from build123d import *

# Parameters (mm, degrees)
SKETCH2_W                        = 1244.6
SKETCH2_H                        = 69.85
BASE_FLANGE1_DEPTH               = 3.2639
EDGE_FLANGE1_STRIP_W             = 15.5956
EDGE_FLANGE1_STRIP_H             = 3.2639
EDGE_FLANGE1_STRIP_CUT_DEPTH     = 1244.6
EDGE_FLANGE1_STRIP_2_W           = 15.5956
EDGE_FLANGE1_STRIP_2_H           = 3.2639
EDGE_FLANGE1_STRIP_CUT_2_DEPTH   = 1244.6
EDGE_FLANGE1_DEPTH               = 1244.6
EDGE_FLANGE1_BEND_DEPTH          = 1244.6
F_10_0_1935_DIAMETER_HOLE1_D     = 4.9149
SKETCH28_R                       = 24.60625
CUT_EXTRUDE1_DEPTH               = 630.738057619
F_10_0_1935_DIAMETER_HOLE5_D     = 4.9149
F_10_0_1935_DIAMETER_HOLE6_D     = 4.9149
F_10_0_1935_DIAMETER_HOLE7_D     = 4.9149
F_25_64_0_39063_DIAMETER_HOLE1_D = 9.922002
F_25_64_0_39063_DIAMETER_HOLE2_D = 9.922002
F_10_0_1935_DIAMETER_HOLE9_D     = 4.9149
LPATTERN1_COUNT                  = 13
LPATTERN1_PITCH                  = 101.6
F_10_0_1935_DIAMETER_HOLE10_D    = 4.9149
F_10_0_1935_DIAMETER_HOLE11_D    = 4.9149
SKETCH69_W                       = 673.1
SKETCH69_H                       = 38.1
SKETCH69_W_2                     = 215.9
CUT_EXTRUDE2_DEPTH               = 630.738057619
FILLET3_R                        = 12.7


# Sheet-metal steps are written as plain solids
with BuildPart() as part:
    # Sketch2 → Base-Flange1 (new body)
    with BuildSketch(Plane.XY):
        Rectangle(SKETCH2_W, SKETCH2_H)
    extrude(amount=-BASE_FLANGE1_DEPTH)

    # Edge-Flange1 strip (across the edge) → Edge-Flange1 strip cut (cut)
    with BuildSketch(Plane(origin=(622.3, 34.925, 0), x_dir=(0, -1, 0), z_dir=(-1, 0, 0))):
        with Locations((-3.2639, -1.63195)):
            Rectangle(EDGE_FLANGE1_STRIP_W, EDGE_FLANGE1_STRIP_H)
    extrude(amount=EDGE_FLANGE1_STRIP_CUT_DEPTH, mode=Mode.SUBTRACT)

    # Edge-Flange1 strip 2 (across the edge) → Edge-Flange1 strip cut 2 (cut)
    with BuildSketch(Plane(origin=(-622.3, -34.925, 0), x_dir=(0, 1, 0), z_dir=(1, 0, 0))):
        with Locations((-3.2639, -1.63195)):
            Rectangle(EDGE_FLANGE1_STRIP_2_W, EDGE_FLANGE1_STRIP_2_H)
    extrude(amount=EDGE_FLANGE1_STRIP_CUT_2_DEPTH, mode=Mode.SUBTRACT)

    # Edge-Flange1 section (across the edge) → Edge-Flange1 (add)
    with BuildSketch(Plane(origin=(622.3, 34.925, 0), x_dir=(0, -1, 0), z_dir=(-1, 0, 0))):
        with BuildLine():
            Line((0, 1.27), (0, 66.5861))
            Line((0, 66.5861), (3.2639, 66.5861))
            Line((3.2639, 66.5861), (3.2639, 1.27))
            ThreePointArc((3.2639, 1.27), (3.635874388, 0.371974388), (4.5339, 0))
            Line((4.5339, 0), (4.5339, -3.2639))
            ThreePointArc((4.5339, -3.2639), (1.327948565, -1.935951435), (0, 1.27))
        make_face()
    extrude(amount=EDGE_FLANGE1_DEPTH)

    # Edge-Flange1 section 2 (across the edge) → Edge-Flange1 bend (add)
    with BuildSketch(Plane(origin=(-622.3, -34.925, 0), x_dir=(0, 1, 0), z_dir=(1, 0, 0))):
        with BuildLine():
            Line((0, 1.27), (0, 66.5861))
            Line((0, 66.5861), (3.2639, 66.5861))
            Line((3.2639, 66.5861), (3.2639, 1.27))
            ThreePointArc((3.2639, 1.27), (3.635874388, 0.371974388), (4.5339, 0))
            Line((4.5339, 0), (4.5339, -3.2639))
            ThreePointArc((4.5339, -3.2639), (1.327948565, -1.935951435), (0, 1.27))
        make_face()
    extrude(amount=EDGE_FLANGE1_BEND_DEPTH)

    # #10 (0.1935) Diameter Hole1 (through all)
    with Locations(Plane(origin=(0, 0, -3.2639), x_dir=(-1, 0, 0), z_dir=(0, 0, -1))):
        with Locations((552.45, 22.225), (603.25, 22.225), (603.25, -22.225), (552.45, -22.225), (501.65, -22.225), (501.65, 22.225)):
            Hole(F_10_0_1935_DIAMETER_HOLE1_D / 2)

    # Sketch28 → Cut-Extrude1 (cut, through all)
    with BuildSketch(Plane.XZ.offset(34.925)):
        with Locations(Location((576.2625, 34.8361, 0), (0, 0, 270))):
            Circle(SKETCH28_R)
    extrude(amount=-CUT_EXTRUDE1_DEPTH, mode=Mode.SUBTRACT)

    # #10 (0.1935) Diameter Hole5 (through all)
    with Locations(Plane(origin=(0, -34.925, 0), x_dir=(-1, 0, 0), z_dir=(0, -1, 0))):
        with Locations((-173.38675, -58.6486), (-173.38675, -11.0236), (-268.63675, -58.6486), (-268.63675, -11.0236)):
            Hole(F_10_0_1935_DIAMETER_HOLE5_D / 2)

    # #10 (0.1935) Diameter Hole6 (through all)
    with Locations(Plane(origin=(0, 0, -3.2639), x_dir=(-1, 0, 0), z_dir=(0, 0, -1))):
        with Locations((-233.71175, 22.225), (-208.31175, 22.225), (-208.31175, -22.225), (-233.71175, -22.225)):
            Hole(F_10_0_1935_DIAMETER_HOLE6_D / 2)

    # #10 (0.1935) Diameter Hole7 (through all)
    with Locations(Plane(origin=(0, 0, -3.2639), x_dir=(-1, 0, 0), z_dir=(0, 0, -1))):
        with Locations((463.55, 0), (368.3, 0)):
            Hole(F_10_0_1935_DIAMETER_HOLE7_D / 2)

    # 25/64 (0.39063) Diameter Hole1 (through all)
    with Locations(Plane(origin=(0, 0, -3.2639), x_dir=(-1, 0, 0), z_dir=(0, 0, -1))):
        with Locations((44.41825, -20.6375), (44.41825, 20.6375)):
            Hole(F_25_64_0_39063_DIAMETER_HOLE1_D / 2)

    # 25/64 (0.39063) Diameter Hole2 (through all)
    with Locations(Plane(origin=(0, 34.925, 0), x_dir=(1, 0, 0), z_dir=(0, 1, 0))):
        with Locations((75.05065, -14.1986), (75.05065, -55.4736)):
            Hole(F_25_64_0_39063_DIAMETER_HOLE2_D / 2)

    # #10 (0.1935) Diameter Hole9 (through all)
    with Locations(Plane(origin=(0, -34.925, 0), x_dir=(-1, 0, 0), z_dir=(0, -1, 0))):
        with Locations((609.6, -12.6111)):
            f_10_0_1935_diameter_hole9 = Hole(F_10_0_1935_DIAMETER_HOLE9_D / 2)

    # LPattern1: #10 (0.1935) Diameter Hole9 ×13, 7 skipped
    with Locations(*[(i * LPATTERN1_PITCH, 0, 0) for i in range(1, LPATTERN1_COUNT) if i not in (1, 3, 5, 7, 8, 10, 12)]):
        add(f_10_0_1935_diameter_hole9, mode=Mode.SUBTRACT)

    # #10 (0.1935) Diameter Hole10 (through all)
    with Locations(Plane(origin=(0, 34.925, 0), x_dir=(1, 0, 0), z_dir=(0, 1, 0))):
        with Locations((612.775, -12.6111), (612.775, -57.0611)):
            Hole(F_10_0_1935_DIAMETER_HOLE10_D / 2)

    # #10 (0.1935) Diameter Hole11 (through all)
    with Locations(Plane(origin=(0, 0, -3.2639), x_dir=(-1, 0, 0), z_dir=(0, 0, -1))):
        with Locations((-612.775, 19.05), (-612.775, -19.05)):
            Hole(F_10_0_1935_DIAMETER_HOLE11_D / 2)

    # Sketch69 → Cut-Extrude2 (cut, through all)
    with BuildSketch(Plane(origin=(0, 34.925, 0), x_dir=(1, 0, 0), z_dir=(0, 1, 0))):
        with Locations((-285.75, -47.5361)):
            Rectangle(SKETCH69_W, SKETCH69_H)
        with Locations((400.05, -47.5361)):
            Rectangle(SKETCH69_W_2, SKETCH69_H)
    extrude(amount=-CUT_EXTRUDE2_DEPTH, mode=Mode.SUBTRACT)

    # Fillet3
    fillet3_edges = [part.edges().sort_by_distance(p)[0] for p in [
        (-622.3, 33.29305, 28.4861),
        (50.8, 33.29305, 66.5861),
        (50.8, 33.29305, 28.4861),
        (-622.3, -33.29305, 28.4861),
        (50.8, -33.29305, 28.4861),
        (50.8, -33.29305, 66.5861),
        (292.1, 33.29305, 28.4861),
        (508, 33.29305, 66.5861),
        (292.1, 33.29305, 66.5861),
        (508, 33.29305, 28.4861),
        (292.1, -33.29305, 66.5861),
        (292.1, -33.29305, 28.4861),
        (508, -33.29305, 28.4861),
        (508, -33.29305, 66.5861),
        (622.3, 33.29305, 66.5861),
        (622.3, -33.29305, 66.5861),
    ]]
    fillet(fillet3_edges, radius=FILLET3_R)


solid = part.part
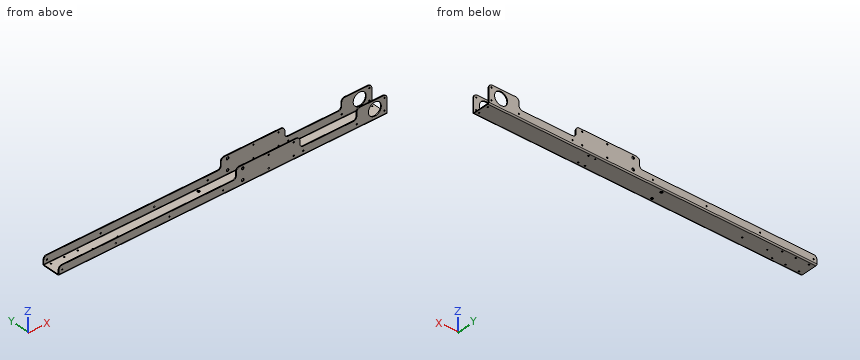
For this review, take the finished solid that the model builds, in its own axes (mm). Round coordinates to 2 decimals unless told otherwise and drop trailing zeros. Write each loop counter-clockwise with the first axis right and the second up, starting at its lowest first coordinate (ties: lowest second). Pieces come first, ordered by that corner, then holes. Notation, with made-up numbers: (69, 74) -> (111, 74) arc R33 cw to (111, 112) -> close; hole circle Ø9 at (46.5, 83). An arc over 180 degrees is marked (long way). Put each result on its own line as item: value.
Q1. To check wall thickness, follow L1, parallel to Y at x = 249, z = 48 (3 decimals); L2, parallel to Z at x = 1, y = 11; L3, parallel to Z at x = -609, y = 33. State the ranges of each line that lie inside material, in increasing order. Write a range as [from, to].
Determined:
L1: y = [-34.925, -31.661], [31.661, 34.925]
L2: z = [-3.26, 0]
L3: z = [-2.44, 10.23], [14.99, 28.49]
Q2. Consider section A-A on x = -131. State the section outline as (y, z) points (3 decimals), and give its area (3 significant figures).
Determined:
outline: (-34.925, 1.27) arc R4.534 ccw to (-30.391, -3.264) -> (30.391, -3.264) arc R4.534 ccw to (34.925, 1.27) -> (34.925, 28.486) -> (31.661, 28.486) -> (31.661, 1.27) arc R1.27 cw to (30.391, 0) -> (-30.391, 0) arc R1.27 cw to (-31.661, 1.27) -> (-31.661, 28.486) -> (-34.925, 28.486) -> close
area: 406 mm^2
Q3. Clearance check with flat-ended pins moving along their axes: pin 1 Ø1 at (y, z) = (-34, 48.5) entering from -X; pin 2 Ø1.5 at (x, y) = (147, -23) entering from +Z. State where each tip first meets the part, or that it passes through.
Determined:
pin 1: stops at x = 50.8
pin 2: stops at z = 0
Q4. Consider section B-B on x = 156.5. State the section outline as (y, z) points (3 decimals), and give its area (3 significant figures).
Determined:
outline: (-34.925, 1.27) arc R4.534 ccw to (-30.391, -3.264) -> (30.391, -3.264) arc R4.534 ccw to (34.925, 1.27) -> (34.925, 66.586) -> (31.661, 66.586) -> (31.661, 1.27) arc R1.27 cw to (30.391, 0) -> (-30.391, 0) arc R1.27 cw to (-31.661, 1.27) -> (-31.661, 66.586) -> (-34.925, 66.586) -> close
area: 655 mm^2
